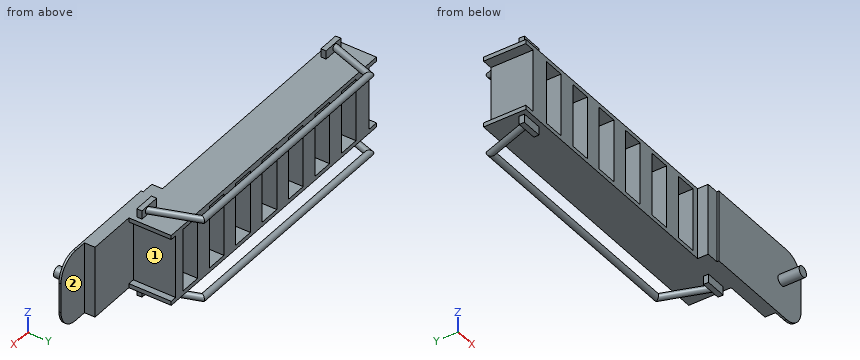
from build123d import *

# Parameters (mm, degrees)
SKETCH1_W                = 140
SKETCH1_H                = 2
BOSS_EXTRUDE3_DEPTH      = 20
SKETCH3_W                = 8
SKETCH3_H                = 20
SKETCH3_W_2              = 9
BOSS_EXTRUDE4_DEPTH      = 30
SKETCH4_W                = 140
SKETCH4_H                = 20
BOSS_EXTRUDE6_DEPTH      = 2
SKETCH6_W                = 30
SKETCH6_H                = 20
CUT_EXTRUDE4_DEPTH       = 3
SKETCH8_W                = 45.941462796
SKETCH8_H                = 34
BOSS_EXTRUDE7_DEPTH      = 5
SKETCH9_W                = 10
SKETCH9_H                = 2.440826928
BOSS_EXTRUDE8_DEPTH      = 4
SWEEP4_PROFILE_R         = 1.5
MIRROR10_COPY_1_SKETCH_W = 10
MIRROR10_COPY_1_SKETCH_H = 2.440826928
MIRROR10_COPY_1_DEPTH    = 4
MIRROR10_COPY_2_SKETCH_R = 1.5
SKETCH75_W               = 56.059600345
SKETCH75_H               = 34
BOSS_EXTRUDE11_DEPTH     = 1
SKETCH84_R               = 2.5
BOSS_EXTRUDE12_DEPTH     = 10
FILLET1_R                = 10


with BuildPart() as part:
    # Sketch1 → Boss-Extrude3 (new body)
    with BuildSketch(Plane(origin=(0, 0, 0), x_dir=(1, 0, 0), z_dir=(0, 1, 0))):
        with Locations((70, 1)):
            Rectangle(SKETCH1_W, SKETCH1_H)
    extrude(amount=BOSS_EXTRUDE3_DEPTH)

    # Sketch3 → Boss-Extrude4 (add)
    with BuildSketch(Plane(origin=(0, 0, -2), x_dir=(-1, 0, 0), z_dir=(0, 0, -1))):
        with Locations((-136, 10)):
            Rectangle(SKETCH3_W, SKETCH3_H)
        with Locations((-118, 10)):
            Rectangle(SKETCH3_W, SKETCH3_H)
        with Locations((-100, 10)):
            Rectangle(SKETCH3_W, SKETCH3_H)
        with Locations((-82, 10)):
            Rectangle(SKETCH3_W, SKETCH3_H)
        with Locations((-64, 10)):
            Rectangle(SKETCH3_W, SKETCH3_H)
        with Locations((-46, 10)):
            Rectangle(SKETCH3_W, SKETCH3_H)
        with Locations((-28, 10)):
            Rectangle(SKETCH3_W, SKETCH3_H)
        with Locations((-9.5, 10)):
            Rectangle(SKETCH3_W_2, SKETCH3_H)
    extrude(amount=BOSS_EXTRUDE4_DEPTH)

    # Sketch4 → Boss-Extrude6 (add)
    with BuildSketch(Plane(origin=(0, 0, -32), x_dir=(-1, 0, 0), z_dir=(0, 0, -1))):
        with Locations((-70, 10)):
            Rectangle(SKETCH4_W, SKETCH4_H)
    extrude(amount=BOSS_EXTRUDE6_DEPTH)

    # Sketch6 → Cut-Extrude4 (cut)
    with BuildSketch(Plane(origin=(140, 0, 0), x_dir=(0, 0, -1), z_dir=(1, 0, 0))):
        with Locations((17, 10)):
            Rectangle(SKETCH6_W, SKETCH6_H)
    extrude(amount=-CUT_EXTRUDE4_DEPTH, mode=Mode.SUBTRACT)

    # Sketch8 → Boss-Extrude7 (add)
    with BuildSketch(Plane.XZ):
        with Locations((140.102979593, -17)):
            Rectangle(SKETCH8_W, SKETCH8_H)
    extrude(amount=BOSS_EXTRUDE7_DEPTH)

    # Sketch9 → Boss-Extrude8 (add)
    with BuildSketch(Plane.XY):
        with Locations((7.209980337, 3.43195512)):
            Rectangle(SKETCH9_W, SKETCH9_H)
    boss_extrude8 = extrude(amount=BOSS_EXTRUDE8_DEPTH)

    # Sweep4: sweep along a path in Sketch35
    with BuildLine(Plane.XY.offset(2)) as sweep4_path:
        Line((5.644054271, 3.447454854), (13.359758823, 25.754529488))
        Line((13.359758823, 25.754529488), (70, 25.754529488))
    # Sweep4 profile (on start of the path) → Sweep4 (sweep)
    with BuildSketch(Plane(origin=(5.644054271, 3.447454854, 2), x_dir=(0.9450642967083543, -0.3268844980832583, 0), z_dir=(0.3268844980832583, 0.9450642967083543, 0))):
        Circle(SWEEP4_PROFILE_R)
    sweep4 = sweep(path=sweep4_path.line, transition=Transition.RIGHT)

    # Mirror9: Boss-Extrude8, Sweep4 across plane
    add(boss_extrude8.mirror(Plane(origin=(70, 0, 0), x_dir=(0, 0, 1), z_dir=(1, 0, 0))))
    add(sweep4.mirror(Plane(origin=(70, 0, 0), x_dir=(0, 0, 1), z_dir=(1, 0, 0))))

    # Mirror10: Boss-Extrude8, Sweep4 across plane
    add(boss_extrude8.mirror(Plane.XY.offset(-17)))
    add(sweep4.mirror(Plane.XY.offset(-17)))

    # Mirror10 copy 1 sketch → Mirror10 copy 1 (add)
    with BuildSketch(Plane(origin=(140, 0, -34), x_dir=(-1, 0, 0), z_dir=(0, 0, -1))):
        with Locations((7.209980337, 3.43195512)):
            Rectangle(MIRROR10_COPY_1_SKETCH_W, MIRROR10_COPY_1_SKETCH_H)
    extrude(amount=MIRROR10_COPY_1_DEPTH)

    # Mirror10 copy 2: sweep along a path in Mirror10 copy 2 path
    with BuildLine(Plane(origin=(140, 0, -36), x_dir=(-1, 0, 0), z_dir=(0, 0, -1))) as mirror10_copy_2_path:
        Line((5.644054271, 3.447454854), (13.359758823, 25.754529488))
        Line((13.359758823, 25.754529488), (70, 25.754529488))
    # Mirror10 copy 2 sketch → Mirror10 copy 2 (sweep)
    with BuildSketch(Plane(origin=(134.355945729, 3.447454854, -36), x_dir=(-0.9450642967083543, -0.3268844980832583, 0), z_dir=(-0.3268844980832583, 0.9450642967083543, 0))):
        Circle(MIRROR10_COPY_2_SKETCH_R)
    sweep(path=mirror10_copy_2_path.line, transition=Transition.RIGHT)

    # Sketch75 → Boss-Extrude11 (add)
    with BuildSketch(Plane.XZ.offset(5)):
        with Locations((151.050400416, -17)):
            Rectangle(SKETCH75_W, SKETCH75_H)
    extrude(amount=BOSS_EXTRUDE11_DEPTH)

    # Sketch84 → Boss-Extrude12 (add)
    with BuildSketch(Plane.XZ.offset(6)):
        with Locations(Location((165.821290963, -17, 0), (0, 0, 270))):
            Circle(SKETCH84_R)
    extrude(amount=BOSS_EXTRUDE12_DEPTH)

    # Fillet1
    fillet1_edges = [part.edges().sort_by_distance(p)[0] for p in [
        (179.080200588, -5.5, -34),
        (179.080200588, -5.5, 0),
    ]]
    fillet(fillet1_edges, radius=FILLET1_R)


solid = part.part
For this review, take the finished solid that the model builds, in its own axes (mm). Face numbers are marked on the shaded views. Round coordinates to 2 decimals unless told otherwise and drop trailing zeros. Write each loop counter-clockwise with the first axis right and the second up, starting at its lowest first coordinate (ties: lowest second). Pieces come first, ordered by that corner, then holes. Notation, with made-up numbers: (49.5, 85) -> (73.5, 85) arc R27 ccw to (73.5, 101) -> close; hole circle Ø7 at (24, -7). An arc over 180 degrees is marked (long way). Put each result on its own line as item: value.
Q1. To check wall thickness, follow L1, parallel to X at y = 4, z = 0.5; L2, parallel to Z at x = 32.5, y = 19.5; L3, parallel to Y at x = 82, z = -32.5. State the ranges of each line that lie inside material, in increasing order. Write a range as [from, to].
Determined:
L1: x = [2.21, 12.21], [127.79, 137.79]
L2: z = [-34, -32], [-2, 0]
L3: y = [0, 20]
Q2. Consider section A-A on x = 36. State the section outline as (y, z) points, and give its area (3 significant figures).
Determined:
outline: (0, -34) -> (20, -34) -> (20, -32) -> (0, -32) -> close; (0, -2) -> (20, -2) -> (20, 0) -> (0, 0) -> close; circle Ø3 at (25.75, -36); circle Ø3 at (25.75, 2)
area: 94.1 mm^2
Q3. Consider section D-D on x = 154.5. State the section outline as (y, z) points, and give its area (3 significant figures).
Determined:
outline: (-6, -34) -> (0, -34) -> (0, 0) -> (-6, 0) -> close
area: 204 mm^2
Q4. Consider section B-B on z = -22. Give the number of separate pieces and of enclosed holes in the cut face, and give its area (3 significant figures).
Determined:
separate pieces: 7
enclosed holes: 0
area: 1,530 mm^2
Q5. Clearance check with flat-ended pins moving along their axes: pin 1 Ø10 at (y, z) = (6.5, -15.5) entering from -X; pin 2 Ø2 at (y, z) = (3, -36.5) entering from -X; pin 3 Ø0.7 at (y, z) = (3, 1) entering from +X. State where each tip first meets the part, or that it passes through.
Determined:
pin 1: stops at x = 5
pin 2: stops at x = 2.21
pin 3: stops at x = 137.79
Q6. The part is to be moulded in two halves that separate along Z. For the marked faces 1 and 2, say which applies: released by +Z, released by -Z, zero draft, split by the parting line, or undercut.
Determined:
face 1: undercut
face 2: zero draft
